Check sheet for the modelled part. Datum: model origin and axes. Units: mm. A direction names the side the tool comes from. Give positions to 0.01 mm unless a question says otherwise; leave off trailing zeros. Loops run counter-clockwise (first coordinate to the right, second up) from the corner with the lowest first, then second, coordinate; pieces in that order, holes last. Notation, with made-up numbers: M 89,2 L 120,2 A10 cw 120,6 Z; hole C 64.5,65 d4. An arc over 180 degrees is marked long. Use one line per item in the form item = value.
from build123d import *

# Parameters (mm, degrees)
EXTRUDE020_DEPTH         = 10
CIRCLE002_R              = 25
EXTRUDE019_DEPTH         = 7
CHAMFER002_SIZE          = 2
CLONE033_ROLL_ANGLE      = 180
CLONE033_PLACEMENT_ANGLE = -90


with BuildPart() as extrude020:
    # Sketch030 (on Face4 of Chamfer002) → Extrude020 (new body, symmetric)
    with BuildSketch(Plane(origin=(0, 7, 0), x_dir=(-1, 0, 0), z_dir=(0, 1, 0))):
        with BuildLine():
            ThreePointArc((3.75, 7.5), (0, 11.25), (-3.75, 7.5))
            Line((-3.75, 7.5), (-3.75, -7.5))
            ThreePointArc((-3.75, -7.5), (0, -11.25), (3.75, -7.5))
            Line((3.75, 7.5), (3.75, -7.5))
        make_face()
    extrude(amount=EXTRUDE020_DEPTH, both=True)


with BuildPart() as lock_right_external:
    # Circle002 → Extrude019 (new body)
    with BuildSketch(Plane.XZ):
        Circle(CIRCLE002_R)
    extrude(amount=-EXTRUDE019_DEPTH)

    # Chamfer002
    chamfer002_edges = [lock_right_external.edges().sort_by_distance(p)[0] for p in [
        (-25, 7, 0),
    ]]
    chamfer(chamfer002_edges, length=CHAMFER002_SIZE)

    # Cut004: cut Extrude020
    add(extrude020.part, mode=Mode.SUBTRACT)


with BuildPart() as lock_right_external_1:
    # Cut004 placement: moved
    add(lock_right_external.part.moved(Location((0, 0, -83.343755))))


with BuildPart() as lock_right_external_2:
    # Clone033 roll: moved
    add(lock_right_external_1.part.rotate(Axis((0, 0, 0), (1, 0, 0)), CLONE033_ROLL_ANGLE))


with BuildPart() as lock_right_external_3:
    # Clone033 placement: moved
    add(lock_right_external_2.part.moved(Location((-400, -215, -133.343755))).rotate(Axis((-400, -215, -133.343755), (0, 0, 1)), CLONE033_PLACEMENT_ANGLE))


with BuildPart() as mirror172:
    # Mirror172: instance of Lock_right_external
    add(lock_right_external_3.part.mirror(Plane(origin=(0, 0, 0), x_dir=(0, -1, 0), z_dir=(1, 0, 0))))


solid = mirror172.part
1) Set-up check for faces 1 (the face through (404, -211.25, -50)), 2 (the face through (400, -220, -50)): record each of +Z, -Z, +X, -X, +Y, -Y from which the full face is reachable in a straight line by a thin tool's end or side.
Evaluation:
face_1 = +X, -X
face_2 = +Z, -Z, -X, +Y, -Y
2) Section check D-D (x = 403.5). Record the cut outline in (y, z).
Evaluation:
outline = C -215,-50 d50; hole M -218.75,-57.5 A3.75 ccw -211.25,-57.5 L -211.25,-42.5 A3.75 ccw -218.75,-42.5 Z
3) Section check A-A (y = -215). Record the cut outline in (x, z).
Evaluation:
outline = M 400,-75 L 405,-75 L 407,-73 L 407,-61.25 L 400,-61.25 Z; M 400,-38.75 L 407,-38.75 L 407,-27 L 405,-25 L 400,-25 Z
4) Release check for a two-part mould opening along Y. For faces 3 (the face through (403.55, -215.08, -38.75)), 4 (the face through (407, -220, -50)), 5 (the face through (402.46, -238.09, -40.42)) record: pulls with the +Y half, pulls with the -Y half, needs draft (parallel to the pull), parting line crosses it, or undercut.
Evaluation:
face_3 = undercut
face_4 = needs draft
face_5 = parting line crosses it
5) Depth check by flat-ended pin: pin 1 Ø3.5 at (x, z) = (405, -51) entering from -Y; pin 2 Ø4 at (x, z) = (401.5, -39.5) entering from -Y; pin 3 Ø1.5 at (x, z) = (402.5, -57) entering from +Y. Enter the tip coordinate at first touch or a pass-through.
Evaluation:
pin_1 = -240
pin_2 = -238.51
pin_3 = -190.79
6) Section check B-B (z = -50). Record the cut outline in (x, y), then the cut area to 4 significant figures.
Evaluation:
outline = M 400,-240 L 405,-240 L 407,-238 L 407,-218.75 L 400,-218.75 Z; M 400,-211.25 L 407,-211.25 L 407,-192 L 405,-190 L 400,-190 Z
area = 293.5 mm^2
7) Section check C-C (x = 406). Record the cut outline in (y, z), then the cut area to 3 significant figures.
Evaluation:
outline = C -215,-50 d48; hole M -218.75,-57.5 A3.75 ccw -211.25,-57.5 L -211.25,-42.5 A3.75 ccw -218.75,-42.5 Z
area = 1,650 mm^2
8) Scan lines: line 1 (Y direction, x = 405, z = -41); line 2 (Z direction, x = 405.75, y = -217); line 3 (Y direction, x = 402, z = -43). Record each from-to range of solid material in increasing order.
Evaluation:
line_1 = -238.32 to -218.44, -211.56 to -191.68
line_2 = -74.17 to -60.67, -39.33 to -25.83
line_3 = -239 to -218.75, -211.25 to -191
